Could you check a few things on this model? Use its own coordinates, in mm. A direction names the side the tool comes from. Round coordinates to 2 decimals unless told otherwise and drop trailing zeros. Write each loop counter-clockwise with the first axis right and the second up, starting at its lowest first coordinate (ties: lowest second). Pieces come first, ordered by that corner, then holes. Notation, with made-up numbers: (6.5, 34.5) -> (37.5, 34.5) arc R27 ccw to (37.5, 71.5) -> close; hole circle Ø10 at (-26, 60). An arc over 180 degrees is marked (long way). Return JSON: item names as keys, results as strings.
from build123d import *

# Parameters (mm, degrees)
SKETCH1_R                = 4
BOSS_EXTRUDE1_DEPTH      = 100
DOME1_FACE_RADIUS        = 4
DOME1_HEIGHT             = 4
SKETCH2_R                = 8
BOSS_EXTRUDE2_DEPTH      = 5
BOSS_EXTRUDE3_DEPTH      = 6
BOSS_EXTRUDE3_DEPTH_BACK = 6


with BuildPart() as part:
    # Sketch1 → Boss-Extrude1 (new body)
    with BuildSketch(Plane(origin=(0, 0, 0), x_dir=(1, 0, 0), z_dir=(0, 1, 0))):
        Circle(SKETCH1_R)
    extrude(amount=BOSS_EXTRUDE1_DEPTH)

    # Dome1: a dome of height H over a round flat face of radius A is a cap of a sphere of radius (A * A + H * H) / (2 * H)
    dome1_r = (DOME1_FACE_RADIUS * DOME1_FACE_RADIUS + DOME1_HEIGHT * DOME1_HEIGHT) / (2 * DOME1_HEIGHT)
    dome1_base = Plane((0, 100, 0), z_dir=(0, 1, 0))
    with Locations(dome1_base.offset(DOME1_HEIGHT - dome1_r)):
        dome1_ball = Sphere(dome1_r, mode=Mode.PRIVATE)
    add(split(dome1_ball, bisect_by=dome1_base, keep=Keep.TOP, mode=Mode.PRIVATE))

    # Sketch2 → Boss-Extrude2 (add)
    with BuildSketch(Plane.XZ):
        Circle(SKETCH2_R)
    extrude(amount=BOSS_EXTRUDE2_DEPTH)

    # Sketch3 → Boss-Extrude3 (add, two sides)
    with BuildSketch(Plane.XY) as boss_extrude3_sk:
        Polygon((-4, 13.165812433), (0, 6.759409677), (4, 13.165812433), (0, 19.572215189), align=None)
    extrude(amount=BOSS_EXTRUDE3_DEPTH)
    extrude(boss_extrude3_sk.sketch, amount=-BOSS_EXTRUDE3_DEPTH_BACK)


solid = part.part
1) Will these pins go through, and if not, where does the flat tip stop? pin 1 Ø2.5 at (x, y) = (-2, 16) entering from -Z; pin 2 Ø5 at (y, z) = (25, -6) entering from +X; pin 3 Ø3 at (y, z) = (79, 4.5) entering from +X.
Return value:
{"pin 1": "z = -6", "pin 2": "x = 1.94", "pin 3": "x = 2.65"}
2) For faces 5 (the face through (-2.42, 15.7, 4.29)), 6 (the face through (0, 13, 6)), 7 (the face through (-4, 0, -2)), which set-ups out of +Z, -Z, +X, -X, +Y, -Y let a thin tool reach every point of the face, with its end or its side?
Return value:
{"face 5": "+Z, -X, +Y", "face 6": "+Z, +X, -X, +Y", "face 7": "none"}
3) I want a section at A-A, the plane y = 9. Please give me the cut outline in (x, z).
Return value:
{"outline": "(-1.4, -6) -> (1.4, -6) -> (1.4, -3.75) arc R4 ccw to (1.4, 3.75) -> (1.4, 6) -> (-1.4, 6) -> (-1.4, 3.75) arc R4 ccw to (-1.4, -3.75) -> close"}
4) I want a section at B-B, the plane z = 1.25. Please give me the cut outline in (x, y).
Return value:
{"outline": "(-7.9, -5) -> (7.9, -5) -> (7.9, 0) -> (3.8, 0) -> (3.8, 12.84) -> (4, 13.17) -> (3.8, 13.49) -> (3.8, 100) arc R3.8 ccw to (-3.8, 100) -> (-3.8, 13.49) -> (-4, 13.17) -> (-3.8, 12.84) -> (-3.8, 0) -> (-7.9, 0) -> close"}
5) Thinking about a two-plate mould opening in Y: for faces 1 (the face through (1.846, 5.028, 3.549)), 2 (the face through (-2.42, 15.7, -4.29)), 3 (the face through (-1.73, -2.46, -7.81)), 4 (the face through (0, -5, 0)), which applies, pulls with the +Y half, pulls with the -Y half, needs draft (parallel to the pull), parting line crosses it, or undercut?
Return value:
{"face 1": "undercut", "face 2": "pulls with the +Y half", "face 3": "needs draft", "face 4": "pulls with the -Y half"}
6) I want a section at D-D, the plane y = 81. Please give me the cut outline in (x, z), and give its area (3 significant figures).
Return value:
{"outline": "circle Ø8 at (0, 0)", "area": "50.3 mm²"}
7) If I drill on probe 1 along Y at (x, z) = (-1, 6.5); probe 2 along X at (y, z) = (68.5, 0.25); probe 3 along Y at (x, z) = (-1.5, -5), over which ranges is the centre line in solid material (lowest first)? Write a range as [from, to].
Return value:
{"probe 1": "[-5, 0]", "probe 2": "[-3.99, 3.99]", "probe 3": "[-5, 0], [9.16, 17.17]"}
8) I want a section at C-C, the plane x = 1.75. Please give me the cut outline in (y, z).
Return value:
{"outline": "(-5, -7.81) -> (0, -7.81) -> (0, -3.6) -> (9.56, -3.6) -> (9.56, -6) -> (16.77, -6) -> (16.77, -3.6) -> (100, -3.6) arc R3.6 ccw to (100, 3.6) -> (16.77, 3.6) -> (16.77, 6) -> (9.56, 6) -> (9.56, 3.6) -> (0, 3.6) -> (0, 7.81) -> (-5, 7.81) -> close"}
